Geometry check sheet. Reference: the model listing, model coordinates, mm. A direction names the side the tool comes from. Give positions to 0.01 mm unless a question says otherwise; leave off trailing zeros. Loops run counter-clockwise (first coordinate to the right, second up) from the corner with the lowest first, then second, coordinate; pieces in that order, holes last. Notation, with made-up numbers: (56.25, 9.5) -> (101.25, 9.5) arc R14 cw to (101.25, 28.5) -> close; hole circle Ø8 at (77.25, 69). An arc over 180 degrees is marked (long way). Answer as a JSON object with one key per item and string values.
Autodesk Inventor part; units mm, degrees
ref_plane "YZ Plane" through (0, 0, 0) normal (1, 0, 0) x (0, 1, 0)
ref_plane "XZ Plane" through (0, 0, 0) normal (0, 1, 0) x (-1, 0, 0)
ref_plane "XY Plane" through (0, 0, 0) normal (0, 0, 1) x (1, 0, 0)
sketch "Sketch1" plane through (0, 0, 0) normal (0, 1, 0) x (-1, 0, 0)
  circle A0 centre (0, 0) radius 17.78
  dimension "d0" = 35.56
extrude "Extrusion1" add sketch "Sketch1" along normal blind 2.54
sketch "Sketch2" plane through (0, 2.54, 0) normal (0, 1, 0) x (1, 0, 0)
  line L0 (0, 0) -> (-13.6144, 0)
  dimension "d3" = 13.6144
hole "Hole1" at (-13.6144, 2.54, 0) direction (0, -1, 0) diameter 3.175 end through all
pattern_circular "Circular Pattern1" count 3 over 360 about axis through (0, 0, 0) along (0, 1, 0) of "Hole1"
sketch "Sketch3" plane through (0, 2.54, 0) normal (0, 1, 0) x (1, 0, 0)
  circle A0 centre (6.8072, -11.7904) radius 1.5875
  line L0 (6.8072, -13.3779) -> (11.9048, -13.3779)
  line L1 (6.8072, -10.2029) -> (15.3383, -10.2029)
  line L2 (15.3383, -10.2029) -> (11.7115, -13.3779)
  circle A1 centre (0, 0) radius 17.78
  circle A2 centre (6.8072, 11.7904) radius 1.5875
  line L3 (6.8072, 10.2029) -> (15.7862, 10.2029)
  line L4 (15.7862, 10.2029) -> (14.1062, 14.4538)
  line L5 (6.8072, 13.3779) -> (14.5314, 13.3779)
  line L6 (11.7115, -13.3779) -> (15.2969, -10.2391)
  circle A3 centre (0, 0) radius 17.78
  point P0 (11.7115, 13.3779)
  point P1 (14.5612, 10.2029)
  point P2 (14.5612, -10.2029)
extrude "Extrusion2" cut sketch "Sketch3" against normal blind 2.54 contours A0 L1 A1 L0 | A1 L3 A2 L5
sketch "Sketch4" plane through (0, 2.54, 0) normal (0, 1, 0) x (1, 0, 0)
  circle A0 centre (0, 0) radius 3.175
  dimension "d16" = 6.35
hole "Hole2" at (0, 2.54, 0) direction (0, -1, 0) diameter 6.35 end through all
sketch "Sketch5" plane through (0, 2.54, 0) normal (0, 1, 0) x (1, 0, 0)
  circle A0 centre (-13.6144, 0) radius 1.5875
  line L0 (-13.6144, -1.5875) -> (17.709, -1.5875)
  arc A1 (14.5612, -10.2029) -> (14.5612, 10.2029) centre (0, 0) ccw
  line L1 (-13.6144, -1.5875) -> (-13.6144, 0)
  line L2 (-13.6144, 0) -> (-13.6144, 1.5931)
  line L3 (-13.6144, 1.5931) -> (17.709, 1.5931)
  line L4 (17.709, 1.5931) -> (17.709, -1.5875)
  circle A2 centre (0, 0) radius 3.175
  line L5 (0, 3.175) -> (17.709, 3.175)
  line L6 (0, -3.175) -> (17.4942, -3.175)
  line L7 (17.4942, -3.175) -> (17.709, -1.5875)
  line L8 (17.709, -1.5875) -> (17.709, 3.175)
  point P0 (17.4942, 3.175)
  point P1 (-2.7496, -1.5875)
  point P2 (-2.7464, 1.5931)
  point P3 (-13.6144, 1.5875)
extrude "Extrusion3" cut sketch "Sketch5" against normal blind 2.54 contours A0 L2 L3 A2 L0 | A2 L3 L4 L0 | L0 L7 L6 A2 | L4 A1 | A1 L7 | A2 L5 A1 L3
sketch "Sketch9" plane through (0, 2.54, 0) normal (0, 1, 0) x (1, 0, 0)
  arc A0 (-13.6144, 1.5875) -> (-13.6144, -1.5875) centre (-13.6144, 0) ccw
  arc A1 (6.8072, 13.3779) -> (6.8072, 10.2029) centre (6.8072, 11.7904) ccw
  line L0 (-13.6144, 0) -> (6.8072, 11.7904)
  arc A2 (6.8072, -10.2029) -> (6.8072, -13.3779) centre (6.8072, -11.7904) ccw
  line L1 (6.8072, 11.7904) -> (6.8072, -11.7904)
  line L2 (6.8072, -11.7904) -> (-13.6144, 0)
  line L3 (-13.6144, 0) -> (-13.6144, 11.7904)
  line L4 (-13.6144, 11.7904) -> (6.8072, 11.7904)
  line L5 (6.8072, -11.7904) -> (-13.6144, -11.7904)
  line L6 (-13.6144, -11.7904) -> (-13.6144, 0)
  circle A3 centre (-3.4036, 11.7904) radius 0.635
  circle A4 centre (-3.4036, -11.7904) radius 0.635
  point P0 (0, 0)
  dimension "d40" = 1.27
hole "Hole5" at (-3.4036, 2.54, -11.7904) at (-3.4036, 2.54, 11.7904) direction (0, -1, 0) diameter 1.905 end through all
properties part number "undertable" material "Stainless Steel AISI 304"
1) Tool access check on faces 1 (the face through (11, 1, 10.203)), 2 (the face through (-3.45, 1.25, 10.84)). Record the directions out of +Z, -Z, +X, -X, +Y, -Y that give a thin tool (end or side, any length) a straight path to the whole face; none if there is none.
Geometry check:
{"face 1": "+X, +Y, -Y", "face 2": "+Y, -Y"}
2) Section check A-A on x = 7.5. Record the cut outline in (y, z) (3 decimals), plus the area to 3 significant figures.
Geometry check:
{"outline": "(0, -16.121) -> (2.54, -16.121) -> (2.54, -13.378) -> (0, -13.378) -> close; (0, -10.203) -> (2.54, -10.203) -> (2.54, -3.175) -> (0, -3.175) -> close; (0, 3.175) -> (2.54, 3.175) -> (2.54, 10.203) -> (0, 10.203) -> close; (0, 13.378) -> (2.54, 13.378) -> (2.54, 16.121) -> (0, 16.121) -> close", "area": "49.6 mm2"}
3) Depth check by flat-ended pin: P1, Ø1.3, axis at x = 5.5, y = 1.5, coming from the +Z side; P2, Ø1, axis at x = 12, y = 1.5, coming from the -Z side; P3, Ø0.8, axis at x = 10, y = 1, coming from the +Z side. Enter the tip coordinate at first touch or a pass-through.
Geometry check:
{"P1": "stops at z = 17.11", "P2": "stops at z = -13.56", "P3": "stops at z = 14.97"}
4) Material ranges on line 1 along Z through (x, y) = (-4, 2.05); line 2 along Z through (x, y) = (9.5, 1.75) (3 decimals); line 3 along Z through (x, y) = (0, 0.95) (3 decimals), recorded low to high. Write a range as from..to.
Geometry check:
{"line 1": "z = -17.32..-12.53, -11.05..-1.59, 1.59..11.05, 12.53..17.32", "line 2": "z = -15.029..-13.378, -10.203..-3.175, 3.175..10.203, 13.378..15.029", "line 3": "z = -17.78..-3.175, 3.175..17.78"}
5) Section check C-C on x = -13. Record the cut outline in (y, z).
Geometry check:
{"outline": "(0, -12.13) -> (2.54, -12.13) -> (2.54, -1.59) -> (0, -1.59) -> close; (0, 1.59) -> (2.54, 1.59) -> (2.54, 12.13) -> (0, 12.13) -> close"}
6) Draft check along Z on faces 3 (the face through (-17.77, 1.25, 0.57)), 4 (the face through (0, 0, -4)), 5 (the face through (5.22, 1.25, 11.83)). Enter one of: pulls with the +Z half, pulls with the -Z half, needs draft (parallel to the pull), parting line crosses it, or undercut.
Geometry check:
{"face 3": "parting line crosses it", "face 4": "needs draft", "face 5": "undercut"}
7) Section check B-B on z = 11.5. Record the cut outline in (x, y).
Geometry check:
{"outline": "(-13.56, 0) -> (-4.31, 0) -> (-4.31, 2.54) -> (-13.56, 2.54) -> close; (-2.5, 0) -> (5.25, 0) -> (5.25, 2.54) -> (-2.5, 2.54) -> close"}
8) Section check D-D on y = 1.3. Count the separate pieces of the cut face and the enclosed holes in it, plus the area to 3 significant figures.
Geometry check:
{"separate pieces": "1", "enclosed holes": "2", "area": "773 mm2"}
